```python
from build123d import *

# Parameters (mm, degrees)
SZKIC2_W                    = 50
SZKIC2_H                    = 53
DODANIE_WYCI_GNI_CIE1_DEPTH = 2
ZAOKR_GLENIE1_R             = 3
SZKIC3_W                    = 50
SZKIC3_H                    = 38
DODANIE_WYCI_GNI_CIE2_DEPTH = 18
SZKIC4_W                    = 34
SZKIC4_H                    = 12.5
DODANIE_WYCI_GNI_CIE3_DEPTH = 16
SZKIC5_R                    = 1.6
DODANIE_WYCI_GNI_CIE4_DEPTH = 2
ZAOKR_GLENIE2_R             = 2


with BuildPart() as part:
    # Szkic2 → Dodanie-wyciągnięcie1 (new body)
    with BuildSketch(Plane(origin=(0, 0, 0), x_dir=(1, 0, 0), z_dir=(0, 1, 0))):
        Rectangle(SZKIC2_W, SZKIC2_H)
        with BuildLine():
            Line((22.6, -17.4), (22.6, -20.6))
            ThreePointArc((22.6, -20.6), (21, -22.2), (19.4, -20.6))
            Line((19.4, -20.6), (19.4, -17.4))
            ThreePointArc((19.4, -17.4), (21, -15.8), (22.6, -17.4))
        make_face(mode=Mode.SUBTRACT)
        with BuildLine():
            Line((-22.6, -17.4), (-22.6, -20.6))
            ThreePointArc((-22.6, -20.6), (-21, -22.2), (-19.4, -20.6))
            Line((-19.4, -20.6), (-19.4, -17.4))
            ThreePointArc((-19.4, -17.4), (-21, -15.8), (-22.6, -17.4))
        make_face(mode=Mode.SUBTRACT)
    extrude(amount=DODANIE_WYCI_GNI_CIE1_DEPTH)

    # Zaokrąglenie1
    zaokr_glenie1_edges = [part.edges().sort_by_distance(p)[0] for p in [
        (25, 1, 26.5),
        (-25, 1, 26.5),
    ]]
    fillet(zaokr_glenie1_edges, radius=ZAOKR_GLENIE1_R)

    # Szkic3 → Dodanie-wyciągnięcie2 (add)
    with BuildSketch(Plane(origin=(0, 2, 0), x_dir=(1, 0, 0), z_dir=(0, 1, 0))):
        with Locations((0, 7.5)):
            Rectangle(SZKIC3_W, SZKIC3_H)
    extrude(amount=DODANIE_WYCI_GNI_CIE2_DEPTH)

    # Szkic4 → Dodanie-wyciągnięcie3 (add)
    with BuildSketch(Plane(origin=(0, 2, 0), x_dir=(1, 0, 0), z_dir=(0, 1, 0))):
        with Locations((0, -17.75)):
            Rectangle(SZKIC4_W, SZKIC4_H)
    extrude(amount=DODANIE_WYCI_GNI_CIE3_DEPTH)

    # Szkic5 → Dodanie-wyciągnięcie4 (add)
    with BuildSketch(Plane(origin=(0, 2, 0), x_dir=(1, 0, 0), z_dir=(0, 1, 0))):
        Polygon((-31.5, 7.5), (-25, 14), (-25, 1), align=None)
        with Locations(Location((-28.5, 7.5, 0), (0, 0, 270))):
            Circle(SZKIC5_R, mode=Mode.SUBTRACT)
    dodanie_wyci_gni_cie4 = extrude(amount=-DODANIE_WYCI_GNI_CIE4_DEPTH)

    # Lustro1: Dodanie-wyciągnięcie4 across plane
    add(dodanie_wyci_gni_cie4.mirror(Plane(origin=(0, 0, 0), x_dir=(0, 0, 1), z_dir=(1, 0, 0))))

    # Zaokrąglenie2
    zaokr_glenie2_edges = [part.edges().sort_by_distance(p)[0] for p in [
        (-31.5, 1, -7.5),
        (31.5, 1, -7.5),
    ]]
    fillet(zaokr_glenie2_edges, radius=ZAOKR_GLENIE2_R)


solid = part.part
```
Can you work these out from the model? Positions are in its coordinate system, mm. A direction names the side the tool comes from. Give positions to 0.01 mm unless a question says otherwise; leave off trailing zeros. Write each loop counter-clockwise with the first axis right and the second up, starting at its lowest first coordinate (ties: lowest second). Pieces come first, ordered by that corner, then holes. Notation, with made-up numbers: (37.25, -38) - (72.25, -38) arc R27 cw to (72.25, -2) - close; hole circle Ø9 at (-22, 53). An arc over 180 degrees is marked (long way). Write item = value, one per line. Start each with the question number.
1. For pin 1 (9 mm diameter, centred on x = -2, y = 15.5, fed in from +Z); pin 2 (6 mm diameter, centred on y = 2.5, z = 7, fed in from +X); pin 3 (2.5 mm diameter, centred on x = 28.5, z = -7.5, fed in from -Y); pin 4 (4 mm diameter, centred on x = -28.5, z = -7.5, fed in from +Y), each with a flat end and sliding along its axis, tell me the tip position at first contact or that it passes through.
2. Imagine slicing it at C-C (y = 3). Please give me the cut outline in (x, z).
3. Please list where these lines run through material, in increasing order: line 1 (X direction, y = 1.15, z = -7.5); line 2 (X direction, y = 5.5, z = -21.5); line 3 (X direction, y = 6, z = 16.5).
4. Imagine slicing it at D-D (x = 2). Please give me the cut outline in (y, z).
5. Imagine slicing it at B-B (z = 18.5). Please give me the cut outline in (x, y), and give its area (3 significant figures).
6. Thinking about a two-plate mould opening in X: for faces 1 (the face through (-21, 1, 22.2)), 2 (the face through (0, 2, 25)), 3 (the face through (-26.914, 1.014, -7.708)), 4 (the face through (-17, 10, 18)), which applies, released by +X, released by -X, zero draft, split by the parting line, or undercut?
7. On a 3-axis mill with a long thin cutter (end or side, diameter ignored), from which of +Z, -Z, +X, -X, +Y, -Y can I reach the whole of each face in a straight line? I mean faces 5 (the face through (26.5, 2, -7.6)), 6 (the face through (19.4, 1, 19)), 7 (the face through (-28, 1, -11)). Say none if no direction works.
8. Imagine slicing it at A-A (x = 28.5). Please give me the cut outline in (y, z).
Worked answers:
q1.pin_1 = 24
q1.pin_2 = 25
q1.pin_3 = through
q1.pin_4 = 2
q2.outline = (-25, -26.5) - (25, -26.5) - (25, 11.5) - (17, 11.5) - (17, 24) - (-17, 24) - (-17, 11.5) - (-25, 11.5) - close
q3.line_1 = -30.67 to -30.1, -26.9 to 26.9, 30.1 to 30.67
q3.line_2 = -25 to 25
q3.line_3 = -17 to 17
q4.outline = (0, -26.5) - (20, -26.5) - (20, 11.5) - (18, 11.5) - (18, 24) - (2, 24) - (2, 26.5) - (0, 26.5) - close
q5.outline = (-25, 0) - (-22.6, 0) - (-22.6, 2) - (-25, 2) - close; (-19.4, 0) - (19.4, 0) - (19.4, 2) - (17, 2) - (17, 18) - (-17, 18) - (-17, 2) - (-19.4, 2) - close; (22.6, 0) - (25, 0) - (25, 2) - (22.6, 2) - close
q5.area = 631 mm2
q6.face_1 = undercut
q6.face_2 = zero draft
q6.face_3 = undercut
q6.face_4 = released by -X
q7.face_5 = +Z, -Z, +X, +Y
q7.face_6 = +Y, -Y
q7.face_7 = -Z, -X, +Y, -Y
q8.outline = (0, -10.5) - (2, -10.5) - (2, -9.1) - (0, -9.1) - close; (0, -5.9) - (2, -5.9) - (2, -4.5) - (0, -4.5) - close
